Part model, mm, in its own coordinate system. A direction names the side the tool comes from. Give positions to 0.01 mm unless a question says otherwise; leave off trailing zeros. Write each loop counter-clockwise with the first axis right and the second up, starting at its lowest first coordinate (ties: lowest second). Pieces come first, ordered by that corner, then holes. Notation, with made-up numbers: M 59.25,25.5 L 94.25,25.5 A24 ccw 94.25,50.5 Z; hole C 56,9.5 d11. An arc over 180 degrees is marked long. Answer as CSV lines item,"result". Start each with the question number.
1) Pin check, flat tips, straight feed: pin 1 Ø1 at (y, z) = (-19, 7) entering from -X; pin 2 Ø12 at (x, y) = (1.5, -14) entering from +Z; pin 3 Ø4 at (x, y) = (1.5, -17.5) entering from -Z. Stop position of each tip, or through.
2) Tool access for faces 1 (the cylindrical face through (-1.172, -19.269, 8.923)), 2 (the flat face through (9, 0, -3)), 3 (the cylindrical face through (12.932, -1.479, -5.362)): list every direction of +Z, -Z, +X, -X, +Y, -Y with a clear straight run to the whole face (end or side of a thin tool).
3) Slice it at A-A, the plane z = 0. Give the cut face in (x, y).
4) Slice it at B-B, the plane x = 0. Give the cut face in (y, z).
5) Wall check: line 1 along Y through (x, z) = (7.5, -5.5); line 2 along X through (y, z) = (-1, -0.5); line 3 along Z through (x, y) = (-6.5, -4). Give the ranges that are in metal, low to high. Write a range as from..to.
6) Slice it at D-D, the plane x = 10. Give the cut face in (y, z), plus the area to 3 significant figures.
7) Slice it at C-C, the plane y = -12. Give the cut face in (x, z), plus the area to 3 significant figures.
```python
from build123d import *

# Parameters (mm, degrees)
F0_R     = 14
F0_R_2   = 9
F1_DEPTH = 3
F2_DEPTH = 27
F3_DEPTH = 2
F4_R     = 3.75
F5_DEPTH = 4
F7_R     = 9
F8_DEPTH = 9


with BuildPart() as f1:
    # F0 (on Front) → F1 (new body)
    with BuildSketch(Plane.XZ):
        Circle(F0_R)
        Circle(F0_R_2, mode=Mode.SUBTRACT)
        Circle(F0_R_2)
    extrude(amount=F1_DEPTH)

    # F0 (on Front) → F2 (join)
    with BuildSketch(Plane.XZ):
        Circle(F0_R_2)
    extrude(amount=F2_DEPTH)

    # F0 (on Front) → F3 (join)
    with BuildSketch(Plane.XZ):
        Circle(F0_R_2)
    extrude(amount=-F3_DEPTH)

    # F4 (on face) → F5 (join)
    with BuildSketch(Plane.XZ.offset(27)):
        Circle(F4_R)
    extrude(amount=F5_DEPTH)

    # F7 (on face) → F8 (join)
    with BuildSketch(Plane.XZ.offset(27)):
        Circle(F7_R)
    extrude(amount=F8_DEPTH)


solid = f1.part
```
Found:
1,pin 1,"x = -6.22"
1,pin 2,"z = 9"
1,pin 3,"z = -9"
2,face 1,"-Y"
2,face 2,"+Y"
2,face 3,"+Y, -Y"
3,outline,"M -14,-3 L -9,-3 L -9,-36 L 9,-36 L 9,-3 L 14,-3 L 14,0 L 9,0 L 9,2 L -9,2 L -9,0 L -14,0 Z"
4,outline,"M -36,-9 L -3,-9 L -3,-14 L 0,-14 L 0,-9 L 2,-9 L 2,9 L 0,9 L 0,14 L -3,14 L -3,9 L -36,9 Z"
5,line 1,"-3..0"
5,line 2,"-13.99..13.99"
5,line 3,"-6.22..6.22"
6,outline,"M -3,-9.8 L 0,-9.8 L 0,9.8 L -3,9.8 Z"
6,area,"58.8 mm²"
7,outline,"C 0,0 d18"
7,area,"254 mm²"
